```python
from build123d import *

# Parameters (mm, degrees)
BOSS_EXTRUDE1_DEPTH = 1.2
FILLET1_R           = 5
FILLET2_R           = 0.8


with BuildPart() as part:
    # Sketch1 → Boss-Extrude1 (new body)
    with BuildSketch(Plane.XY):
        with BuildLine():
            Line((-10.5, 0), (-12.5, -2))
            Line((-12.5, -2), (-12, -12))
            Line((-12, -12), (-12.5, -14))
            Line((-12.5, -14), (-14.5, -14))
            Line((-14.5, -14), (-14.5, 3))
            Line((-14.5, 3), (-12.5, 3))
            Line((-12.5, 3), (12.5, 3))
            Line((12.5, 3), (14.5, 3))
            Line((14.5, 3), (14.5, -14))
            Line((14.5, -14), (12.5, -14))
            Line((12.5, -14), (12, -12))
            Line((12, -12), (12.5, -2))
            Line((12.5, -2), (10.5, 0))
            Line((10.5, 0), (8, 0))
            Line((8, 0), (8, -12))
            Line((8, -12), (3.5, -12))
            Line((3.5, -12), (3.5, -6.5))
            ThreePointArc((3.5, -6.5), (0, -3), (-3.5, -6.5))
            Line((-3.5, -6.5), (-3.5, -12))
            Line((-3.5, -12), (-8, -12))
            Line((-8, -12), (-8, 0))
            Line((-8, 0), (-10.5, 0))
        make_face()
    extrude(amount=BOSS_EXTRUDE1_DEPTH)

    # Fillet1
    fillet1_edges = [part.edges().sort_by_distance(p)[0] for p in [
        (-12, -12, 0.6),
        (12, -12, 0.6),
    ]]
    fillet(fillet1_edges, radius=FILLET1_R)

    # Fillet2
    fillet2_edges = [part.edges().sort_by_distance(p)[0] for p in [
        (-12.5, -14, 0.6),
        (-14.5, -14, 0.6),
        (-14.5, 3, 0.6),
        (14.5, 3, 0.6),
        (14.5, -14, 0.6),
        (12.5, -14, 0.6),
        (8, -12, 0.6),
        (3.5, -12, 0.6),
        (-3.5, -12, 0.6),
        (-8, -12, 0.6),
    ]]
    fillet(fillet2_edges, radius=FILLET2_R)


solid = part.part
```
Model file for the job. Use its own axes, mm. A direction names the side the tool comes from. Round coordinates to 2 decimals unless told otherwise and drop trailing zeros. Write each loop counter-clockwise with the first axis right and the second up, starting at its lowest first coordinate (ties: lowest second). Pieces come first, ordered by that corner, then holes. Notation, with made-up numbers: (72.25, -34) - (107.25, -34) arc R19 ccw to (107.25, -15) - close; hole circle Ø1 at (4, -23.5). An arc over 180 degrees is marked (long way). Use CSV: the item, a comma, the result in double quotes. Start each with the question number.
Item 1: Band-saw the part on A-A (y = -1). Write the cut outline in (x, z), and give its area (3 significant figures).
Item 2: Band-saw the part on D-D (x = 0). Write the cut outline in (y, z).
Item 3: Pin check, flat tip, straight feed: P1, Ø0.6, axis at x = 6, z = 1, coming from the -Y side. Stop position of the tip, or through.
Item 4: Tool access for faces 1 (the face through (-6, -12, 1)), 2 (the face through (14.5, -5, 1)), 3 (the face through (12.265, -6.694, 0.592)): list every direction of +Z, -Z, +X, -X, +Y, -Y with a clear straight run to the whole face (end or side of a thin tool).
Item 5: Two-plate mould, pull along X, no slides. Class faces 4 (the face through (0, -2, 1.2)), 5 (the face through (7.76, -11.77, 0.61)), 6 (the face through (14.26, 2.77, 0.61)), 7 (the face through (-14.5, -6, 1)): released by +X, released by -X, zero draft, split by the parting line, or undercut.
Item 6: Drill centre lines: L1, parallel to X at y = -11.25, z = 0.65; L2, parallel to X at y = -2.75, z = 0.7; L3, parallel to X at y = -7.75, z = 0.8. Where is each one in solid material? Low to high. Write a range as [from, to].
Item 7: Band-saw the part on B-B (y = -10). Write the cut outline in (x, z), and give its area (3 significant figures).
Checked values:
1,outline,"(-14.5, 0) - (-11.5, 0) - (-11.5, 1.2) - (-14.5, 1.2) - close; (-8, 0) - (8, 0) - (8, 1.2) - (-8, 1.2) - close; (11.5, 0) - (14.5, 0) - (14.5, 1.2) - (11.5, 1.2) - close"
1,area,"26.4 mm²"
2,outline,"(-3, 0) - (3, 0) - (3, 1.2) - (-3, 1.2) - close"
3,P1,"stops at y = -12"
4,face 1,"+Z, -Z, -Y"
4,face 2,"+Z, -Z, +X, +Y, -Y"
4,face 3,"+Z, -Z"
5,face 4,"zero draft"
5,face 5,"undercut"
5,face 6,"released by +X"
5,face 7,"released by -X"
6,L1,"x = [-14.5, -12.04], [-8, -3.5], [3.5, 8], [12.04, 14.5]"
6,L2,"x = [-14.5, -12.46], [-8, 8], [12.46, 14.5]"
6,L3,"x = [-14.5, -12.21], [-8, -3.5], [3.5, 8], [12.21, 14.5]"
7,outline,"(-14.5, 0) - (-12.1, 0) - (-12.1, 1.2) - (-14.5, 1.2) - close; (-8, 0) - (-3.5, 0) - (-3.5, 1.2) - (-8, 1.2) - close; (3.5, 0) - (8, 0) - (8, 1.2) - (3.5, 1.2) - close; (12.1, 0) - (14.5, 0) - (14.5, 1.2) - (12.1, 1.2) - close"
7,area,"16.6 mm²"
